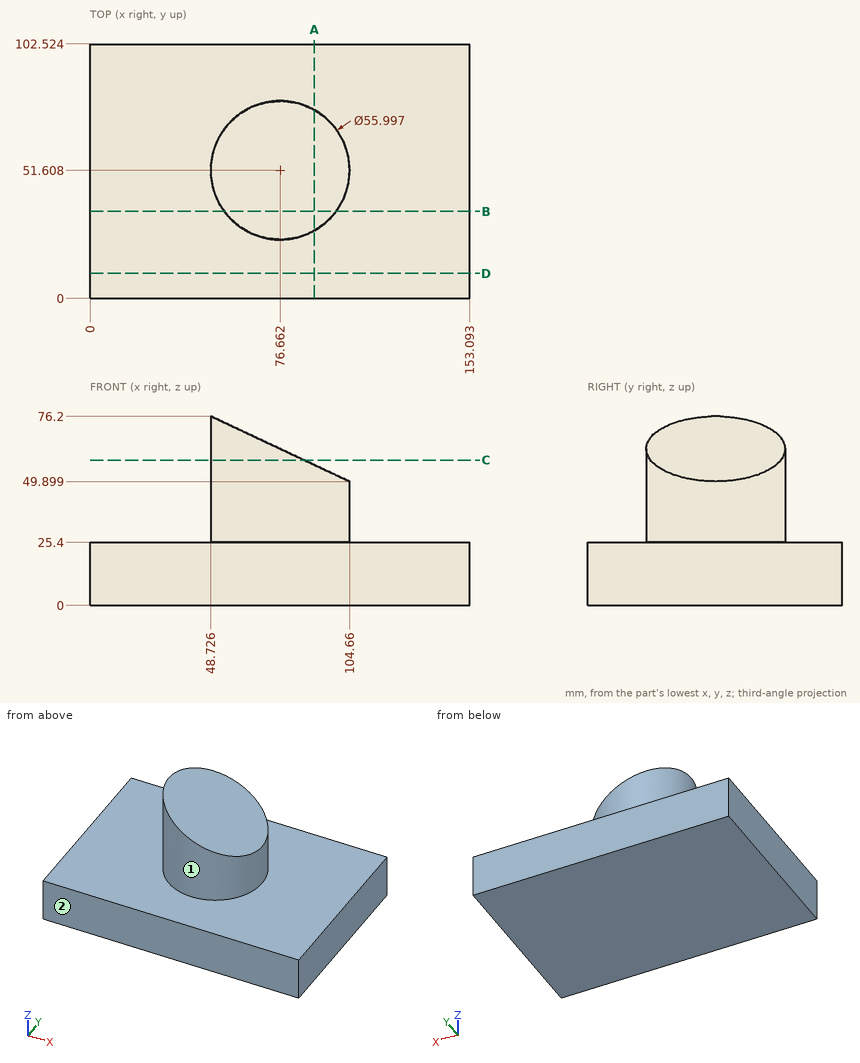
Design review of the part shown in the three views and the two pictorial views. Dimensions are in mm from the part's minimum x, y and z. A direction names the side the tool comes from. Round coordinates to 2 decimals unless told otherwise and drop trailing zeros. Order: outer loops, then holes, each group sorted by start corner. A loop starts at its lowest first (then second) coordinate and runs counter-clockwise, first axis right, second up. Notation, with made-up numbers: (32.5, 61.25) - (58.5, 61.25) arc R29 ccw to (58.5, 93.25) - close; hole circle Ø10 at (36, 9.5). An arc over 180 degrees is marked (long way). Answer in a Markdown table with one row per item.
(1) Take a section at A-A on x = 90.5. Write out the cut boundary in (y, z).
Result set:
| item | result |
|---|---|
| outline | (0, 0) - (102.52, 0) - (102.52, 25.4) - (75.95, 25.4) - (75.95, 56.56) - (27.27, 56.56) - (27.27, 25.4) - (0, 25.4) - close |
(2) Take a section at B-B on y = 35. Write out the cut boundary in (x, z) (1 decimal), plus the area to 3 significant figures.
Result set:
| item | result |
|---|---|
| outline | (0, 0) - (153.1, 0) - (153.1, 25.4) - (99.2, 25.4) - (99.2, 52.5) - (54.1, 73.7) - (54.1, 25.4) - (0, 25.4) - close |
| area | 5,590 mm2 |
(3) Clearance check with flat-ended pins moving along their axes: P1, Ø6, axis at x = 99, y = 61, coming from the +Z side; P2, Ø3, axis at y = 36.5, z = 27.5, coming from the -X side; P3, Ø4, axis at y = 44, z = 48.5, coming from the -X side. State where each tip first meets the part, or that it passes through.
Result set:
| item | result |
|---|---|
| P1 | stops at z = 53.97 |
| P2 | stops at x = 52.19 |
| P3 | stops at x = 49.23 |
(4) Take a section at C-C on z = 58.5. Write out the cut boundary in (x, y).
Result set:
| item | result |
|---|---|
| outline | (86.37, 25.35) - (86.37, 77.87) arc R28 ccw (long way) to start |
(5) Machinability: for the marked faces 1 and 2, which of the approach directions +Z, -Z, +X, -X, +Y, -Y give a long, thin tool a straight path to every point of the face, cutting with its end or side? Answer none if there is none.
Result set:
| item | result |
|---|---|
| face 1 | +Z |
| face 2 | +Z, -Z, +X, -X, -Y |
(6) For line 1 (Z direction, x = 147.5, y = 33); line 2 (X direction, y = 52, z = 35); line 3 (Z direction, x = 66.5, y = 44), list the stretches that pass through material, from the lowest coordinate up. Write a range as from..to.
Result set:
| item | result |
|---|---|
| line 1 | z = 0..25.4 |
| line 2 | x = 48.67..104.66 |
| line 3 | z = 0..67.84 |
(7) Take a section at D-D on y = 10. Write out the cut boundary in (x, z).
Result set:
| item | result |
|---|---|
| outline | (0, 0) - (153.09, 0) - (153.09, 25.4) - (0, 25.4) - close |
